Build history of the part. All positions in model axes, mm. Give positions to 0.01 mm unless a question says otherwise; leave off trailing zeros. Write each loop counter-clockwise with the first axis right and the second up, starting at its lowest first coordinate (ties: lowest second). Pieces come first, ordered by that corner, then holes. Notation, with made-up numbers: (47.25, -35.5) -> (77.25, -35.5) arc R22 cw to (77.25, -10.5) -> close; hole circle Ø9 at (2.25, -33.5). An arc over 180 degrees is marked (long way). One line per question, with ' | ' between items. Start each with the question number.
(1) Drill centre lines: probe 1 along Y at (x, z) = (-55.5, 2.5); probe 2 along X at (y, z) = (12, 5); probe 3 along X at (y, z) = (19.5, 4). Where is each one in solid material? Low to high. Write a range as from..to.
(2) Band-saw the part on C-C, the plane y = 42. Give the cut face in (x, z).
(3) Band-saw the part on A-A, the plane z = 1.25. Give the cut face in (x, y).
(4) Band-saw the part on B-B, the plane x = -4. Give the cut face in (y, z).
from build123d import *

# Parameters (mm, degrees)
EXTRUDE_DEPTH = 10
BOX_W         = 220
BOX_H         = 92
BOX_DEPTH     = 8


with BuildPart() as extrude_body:
    # Sketch001 → Extrude (new body)
    with BuildSketch(Plane.XY):
        Polygon((-95, 0), (95, 0), (85, 61), (-85, 61), align=None)
    extrude(amount=EXTRUDE_DEPTH)


with BuildPart() as obj1:
    # Box → Box (new body)
    with BuildSketch(Plane(origin=(-110, -15, 0), x_dir=(1, 0, 0), z_dir=(0, 0, 1))):
        with Locations((110, 46)):
            Rectangle(BOX_W, BOX_H)
    extrude(amount=BOX_DEPTH)

    # Cut: cut Extrude body
    add(extrude_body.part, mode=Mode.SUBTRACT)


solid = obj1.part
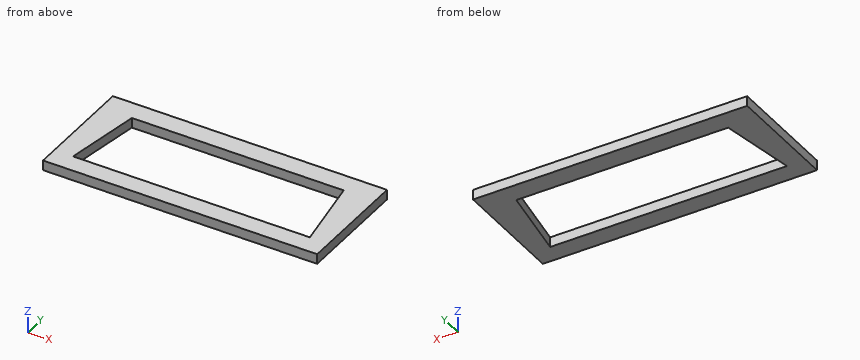
Results:
1) probe 1: y = -15..0, 61..77 | probe 2: x = -110..-93.03, 93.03..110 | probe 3: x = -110..-91.8, 91.8..110
2) outline: (-110, 0) -> (-88.11, 0) -> (-88.11, 8) -> (-110, 8) -> close; (88.11, 0) -> (110, 0) -> (110, 8) -> (88.11, 8) -> close
3) outline: (-110, -15) -> (110, -15) -> (110, 77) -> (-110, 77) -> close; hole (-95, 0) -> (95, 0) -> (85, 61) -> (-85, 61) -> close
4) outline: (-15, 0) -> (0, 0) -> (0, 8) -> (-15, 8) -> close; (61, 0) -> (77, 0) -> (77, 8) -> (61, 8) -> close
